Source: CAD feature listing. Evaluate the final solid. Frame: model axes, mm. A direction names the side the tool comes from. Round coordinates to 2 decimals unless told otherwise and drop trailing zeros. Order: outer loops, then holes, each group sorted by start corner. A loop starts at its lowest first (then second) coordinate and runs counter-clockwise, first axis right, second up.
```python
from build123d import *


with BuildPart() as part:
    # Skizze2 → Rotation1 (revolve)
    with BuildSketch(Plane.XY, mode=Mode.PRIVATE) as rotation1_sk:
        with BuildLine():
            Line((8.75, 20.25), (11.5, 20.25))
            Line((11.5, 20.25), (11.5, -13.5))
            Line((11.5, -13.5), (12.5, -13.5))
            Line((12.5, -13.5), (12.5, -5.5))
            Line((12.5, -5.5), (15.5, -5.5))
            Line((15.5, -5.5), (15.5, 0))
            Line((15.5, 0), (12.5, 0))
            Line((12.5, 0), (12.5, 4))
            Line((12.5, 4), (15.5, 4))
            Line((15.5, 4), (15.5, 20.25))
            ThreePointArc((15.5, 20.25), (13.522970773, 25.022970773), (8.75, 27))
            Line((8.75, 27), (8.75, 20.25))
        make_face()
    revolve(rotation1_sk.sketch.rotate(Axis((0, 275.175103998, 0), (0, -1, 0)), 180), axis=Axis((0, 275.175103998, 0), (0, -1, 0)))


solid = part.part
```
1. First-contact query: pin 1 (10 mm diameter, centred on x = 4, z = 6.5, fed in from -Y); pin 2 (8 mm diameter, centred on x = -4.5, y = -8, fed in from +Z); pin 3 (12 mm diameter, centred on x = 9.5, y = 7, fed in from +Z); pin 4 (1 mm diameter, centred on x = -4.5, y = -3.5, fed in from +Z) (3 decimals). Flat tips, straight axial feed; report the tip coordinate or a pass-through.
2. Section D-D on y = -8. Return loops of the section in (x, z), plus the area to 3 significant figures.
3. Line query: line 1 along Z through (x, y) = (0, 1.5); line 2 along Y through (x, z) = (-8, 4); line 3 along Z through (x, y) = (0, 25.75). Output: solid intervals per line, ascending.
4. Section C-C on y = -3. Return loops of the section in (x, z), plus the area to 3 significant figures.
5. Section A-A on x = 0. Return loops of the section in (y, z), plus the area to 3 significant figures.
6. Section B-B on z = 0. Return loops of the section in (x, y).
7. Pull-direction query (X, two-part tool) for faces 1 (the face through (1.9, 23.58, 8.54)), 2 (the face through (1.5, 3.1, -11.4)), 3 (the face through (2.018, -2.712, -15.368)), 4 (the face through (-1, 0, -13)); classes: released by +X, released by -X, zero draft, split by the parting line, or undercut.
8. Access query for faces 5 (the face through (2.018, 12.239, -15.368)), 6 (the face through (-11.923, 2.028, -3.755)), 7 (the face through (-2, 20.25, -9)). Directions: +Z, -Z, +X, -X, +Y, -Y. A direction counts if a zero-diameter tool reaches every point of the face in a straight line with its end or side. Return the directions, or none.
Result:
1. pin 1: stops at y = -13.5
1. pin 2: stops at z = 15.44
1. pin 3: stops at z = 15.1
1. pin 4: stops at z = 14.975
2. outline: circle Ø25 at (0, 0); hole circle Ø23 at (0, 0)
2. area: 75.4 mm2
3. line 1: z = -12.5 to -11.5, 11.5 to 12.5
3. line 2: y = 20.25 to 27
3. line 3: z = -12.66 to -8.75, 8.75 to 12.66
4. outline: circle Ø31 at (0, 0); hole circle Ø23 at (0, 0)
4. area: 339 mm2
5. outline: (-13.5, -12.5) - (-5.5, -12.5) - (-5.5, -15.5) - (0, -15.5) - (0, -12.5) - (4, -12.5) - (4, -15.5) - (20.25, -15.5) arc R6.75 ccw to (27, -8.75) - (20.25, -8.75) - (20.25, -11.5) - (-13.5, -11.5) - close; (-13.5, 11.5) - (20.25, 11.5) - (20.25, 8.75) - (27, 8.75) arc R6.75 ccw to (20.25, 15.5) - (4, 15.5) - (4, 12.5) - (0, 12.5) - (0, 15.5) - (-5.5, 15.5) - (-5.5, 12.5) - (-13.5, 12.5) - close
5. area: 270 mm2
6. outline: (-15.5, -5.5) - (-12.5, -5.5) - (-12.5, -13.5) - (-11.5, -13.5) - (-11.5, 20.25) - (-8.75, 20.25) - (-8.75, 27) arc R6.75 ccw to (-15.5, 20.25) - (-15.5, 4) - (-12.5, 4) - (-12.5, 0) - (-15.5, 0) - close; (8.75, 20.25) - (11.5, 20.25) - (11.5, -13.5) - (12.5, -13.5) - (12.5, -5.5) - (15.5, -5.5) - (15.5, 0) - (12.5, 0) - (12.5, 4) - (15.5, 4) - (15.5, 20.25) arc R6.75 ccw to (8.75, 27) - close
7. face 1: undercut
7. face 2: undercut
7. face 3: split by the parting line
7. face 4: zero draft
8. face 5: +Y, -Y
8. face 6: none
8. face 7: -Y
